Can you work these out from the drawing? Everything is in mm from the part's minimum corner. A direction names the side the tool comes from. Round coordinates to 2 decimals unless told otherwise and drop trailing zeros. Order: outer loops, then holes, each group sorted by start corner. A loop starts at its lowest first (then second) coordinate and runs counter-clockwise, first axis right, second up. Notation, with made-up numbers: M 31.5,9.25 L 47.5,9.25 A20 ccw 47.5,28.25 Z; hole C 65.5,4.25 d6. An arc over 180 degrees is marked long. Write each question's results on one line, items separated by ' | '. Start each with the question number.
1. Suppose I cut it at A-A on x = 8.5. Write out the boundary of the cut face in (y, z), and give its area (3 significant figures).
2. Please list where these lines run through material, in increasing order: L1, parallel to Z at x = 1.75, y = 9.5; L2, parallel to Y at x = 3.5, z = 20.5 (1 decimal); L3, parallel to Y at x = 2.75, z = 17.75.
3. Suppose I cut it at C-C on y = 12.25. Write out the boundary of the cut face in (x, z), and give its area (3 significant figures).
4. I'm going to push flat-ended pins straight in: pin 1 (1.5 mm diameter, centred on y = 3.5, z = 19.5, fed in from -X); pin 2 (4 mm diameter, centred on y = 8, z = 21, fed in from -X). Where does each tip first touch, or does it pass through?
5. Suppose I cut it at B-B on z = 10.5. Write out the boundary of the cut face in (x, y).
6. For the marked faces 1, 2 and 3, which set-ups out of +Z, -Z, +X, -X, +Y, -Y let a thin tool reach every point of the face, with its end or its side?
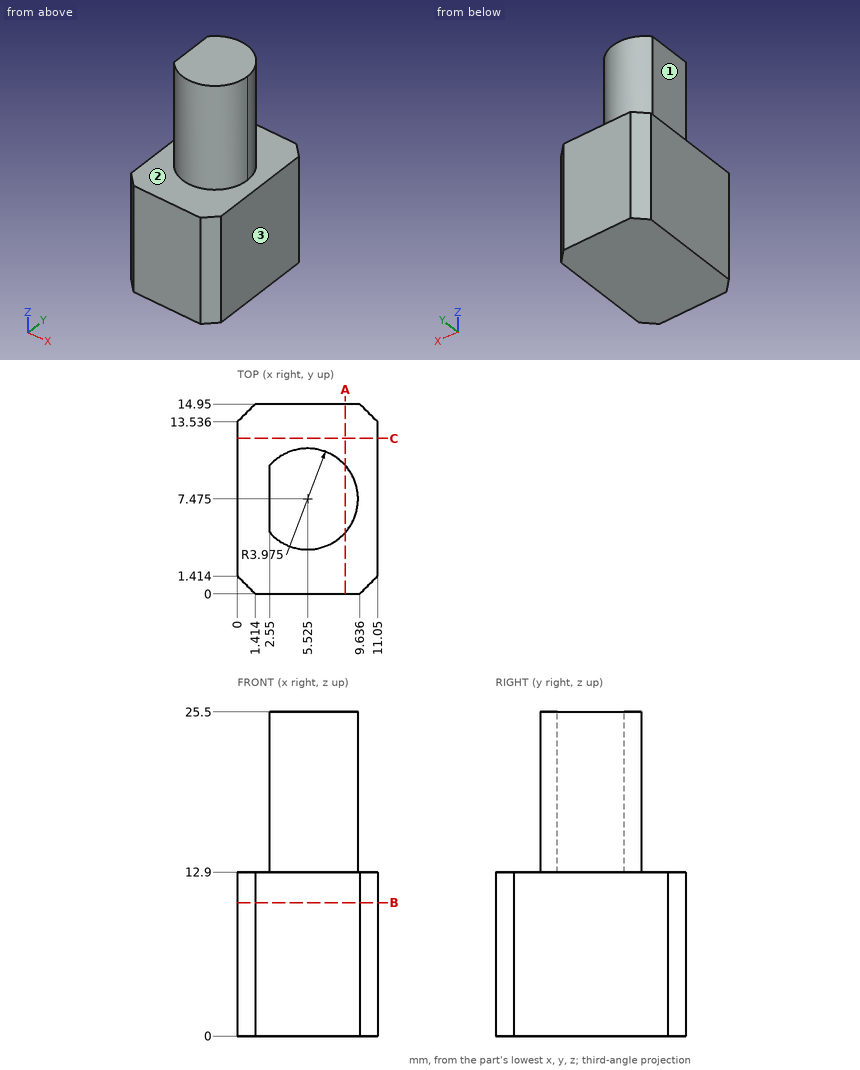
Filled sheet:
1) outline: M 0,0 L 14.95,0 L 14.95,12.9 L 10.11,12.9 L 10.11,25.5 L 4.84,25.5 L 4.84,12.9 L 0,12.9 Z | area: 259 mm^2
2) L1: z = 0 to 12.9 | L2: y = 4.1 to 10.9 | L3: y = 4.63 to 10.32
3) outline: M 0,0 L 11.05,0 L 11.05,12.9 L 0,12.9 Z | area: 143 mm^2
4) pin 1: stops at x = 3.2 | pin 2: stops at x = 2.55
5) outline: M 0,1.41 L 1.41,0 L 9.64,0 L 11.05,1.41 L 11.05,13.54 L 9.64,14.95 L 1.41,14.95 L 0,13.54 Z
6) face 1: +Z, -X, +Y, -Y | face 2: +Z | face 3: +Z, -Z, +X, +Y, -Y
